```python
from build123d import *

# Parameters (mm, degrees)
SKETCH1_R           = 5
SKETCH1_R_2         = 1
BOSS_EXTRUDE1_DEPTH = 6.5
SKETCH5_W           = 2
SKETCH5_H           = 14.476636654


with BuildPart() as part:
    # Sketch1 → Boss-Extrude1 (new body)
    with BuildSketch(Plane.XY):
        with BuildLine():
            Line((13.913051744, -4), (5.285881411, -1.519690003))
            ThreePointArc((5.285881411, -1.519690003), (5.446207293, -0.767350063), (5.5, 0))
            Line((5.5, 0), (4, 8))
            ThreePointArc((4, 8), (0, 12), (-4, 8))
            Line((-4, 8), (-5.5, 0))
            ThreePointArc((-5.5, 0), (-5.446207293, -0.767350063), (-5.285881411, -1.519690003))
            Line((-5.285881411, -1.519690003), (-13.913051744, -4))
            ThreePointArc((-13.913051744, -4), (0, -14.476636654), (13.913051744, -4))
        make_face()
        with Locations(Location((0, 0, 0), (0, 0, 180))):
            Circle(SKETCH1_R, mode=Mode.SUBTRACT)
        with Locations(Location((0, 8, 0), (0, 0, 180))):
            Circle(SKETCH1_R_2, mode=Mode.SUBTRACT)
    extrude(amount=BOSS_EXTRUDE1_DEPTH)

    # Sketch5 → Ø4.0 (4) Diameter Hole1 (revolve, cut)
    with BuildSketch(Plane(origin=(0, 0, 3.25), x_dir=(0, 0, 1), z_dir=(1, 0, 0))):
        with Locations((1, 7.238318327)):
            Rectangle(SKETCH5_W, SKETCH5_H)
    revolve(axis=Axis((0, 6.35, 3.25), (0, -1, 0)), mode=Mode.SUBTRACT)


solid = part.part
```
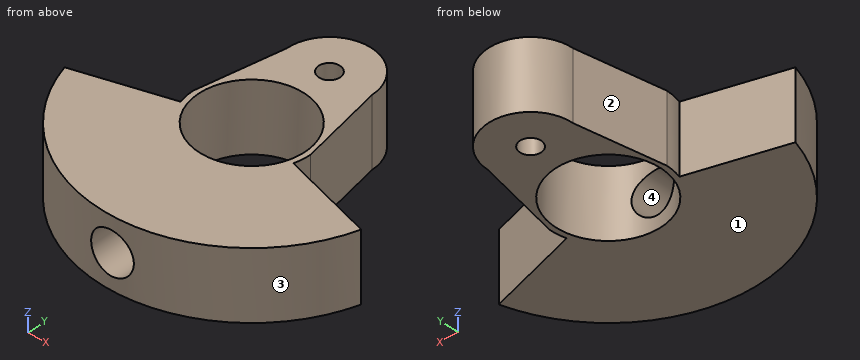
Geometry: final body of the model. Coordinates: model frame, mm. Face numbers are marked on the shaded views. Coordinates: 2 decimals unless noted, no trailing zeros. Loops run counter-clockwise (first coordinate to the right, second up) from the corner with the lowest first, then second, coordinate; pieces in that order, holes last. Notation, with made-up numbers: M -39.75,-34.5 L -29.75,-34.5 A32 cw -29.75,4.5 Z; hole C 31.25,24.5 d8. An arc over 180 degrees is marked long. Put each result on its own line as item: value.
(1) Cut plane B-B on z = 6. Return the cut outline in (x, y).
Answer sheet:
outline: M -13.91,-4 A14.48 ccw 13.91,-4 L 5.29,-1.52 A5.5 ccw 5.5,0 L 4,8 A4 ccw -4,8 L -5.5,0 A5.5 ccw -5.29,-1.52 Z; hole C 0,0 d10; hole C 0,8 d2
(2) First-contact query: pin 1 (1.5 mm diameter, centred on x = -6.5, z = 1, fed in from +Y); pin 2 (1.5 mm diameter, centred on x = 7.5, z = 4, fed in from -Y). Flat tips, straight axial feed; report the tip coordinate or a pass-through.
Answer sheet:
pin 1: stops at y = -1.65
pin 2: stops at y = -12.81
(3) Cut plane A-A on x = 0. Return the cut outline in (y, z).
Answer sheet:
outline: M -14.48,0 L -5,0 L -5,1.25 L -14.48,1.25 Z; M -14.48,5.25 L -5,5.25 L -5,6.5 L -14.48,6.5 Z; M 5,0 L 7,0 L 7,6.5 L 5,6.5 Z; M 9,0 L 12,0 L 12,6.5 L 9,6.5 Z
(4) Draft query along X for the marked faces 1, 2, 3 and 4. Return one class per face: pulls with the +X half, pulls with the -X half, needs draft (parallel to the pull), parting line crosses it, or undercut.
Answer sheet:
face 1: needs draft
face 2: pulls with the -X half
face 3: parting line crosses it
face 4: undercut
(5) Cut plane D-D on y = 3.5. Return the cut outline in (x, z).
Answer sheet:
outline: M -4.84,0 L -3.57,0 L -3.57,6.5 L -4.84,6.5 Z; M 3.57,0 L 4.84,0 L 4.84,6.5 L 3.57,6.5 Z
(6) Cut plane C-C on x = -4.5. Return the cut outline in (y, z).
Answer sheet:
outline: M -13.76,0 L -2.18,0 L -2.18,6.5 L -13.76,6.5 Z; M 2.18,0 L 5.33,0 L 5.33,6.5 L 2.18,6.5 Z
(7) Material intervals for probe 1 along X at (y, z) = (8, 4); probe 2 along Y at (x, z) = (0, 3.75); probe 3 along X at (y, z) = (7.5, 4.75), sorted ascending.
Answer sheet:
probe 1: x = -4 to -1, 1 to 4
probe 2: y = 5 to 7, 9 to 12
probe 3: x = -4.09 to -0.87, 0.87 to 4.09
